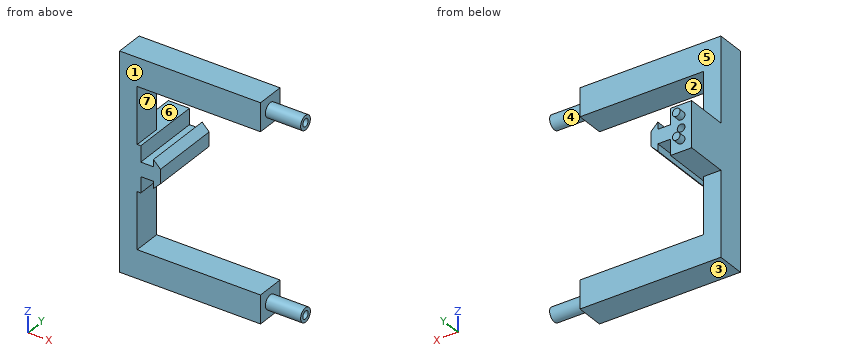
Autodesk Inventor part; units mm, degrees
ref_plane "YZ Plane" through (0, 0, 0) normal (1, 0, 0) x (0, 1, 0)
ref_plane "XZ Plane" through (0, 0, 0) normal (0, 1, 0) x (-1, 0, 0)
ref_plane "XY Plane" through (0, 0, 0) normal (0, 0, 1) x (1, 0, 0)
sketch "Sketch1" plane through (0, 0, 0) normal (0, 1, 0) x (-1, 0, 0)
  line L0 (0, 0) -> (7.62, 0)
  line L1 (7.62, 0) -> (7.62, -16.51)
  line L2 (7.62, -16.51) -> (0, -16.51)
  line L3 (0, -16.51) -> (0, 0)
  line L4 (0, 0) -> (0, -5.715)
  line L5 (0, -5.715) -> (-7.112, -5.715)
  line L6 (-7.112, -5.715) -> (-7.112, -10.795)
  line L7 (-7.112, -10.795) -> (0, -10.795)
  line L8 (-7.112, -5.715) -> (-4.572, -5.715)
  line L9 (-4.572, -5.715) -> (-4.572, -3.175)
  line L10 (-4.572, -3.175) -> (-7.112, -5.715)
  line L11 (-7.112, -10.795) -> (-4.572, -10.795)
  line L12 (-4.572, -10.795) -> (-4.572, -13.335)
  line L13 (-4.572, -13.335) -> (-7.112, -10.795)
  dimension "d0" = 7.62
  dimension "d1" = 16.51
  dimension "d2" = 5.715
  dimension "d3" = 7.112
  dimension "d4" = 5.08
  dimension "d5" = 2.54
  dimension "d6" = 2.54
  dimension "d7" = 2.54
extrude "Extrusion1" add sketch "Sketch1" along normal blind 25.4
sketch "Sketch2" plane through (0, 25.4, 0) normal (0, 1, 0) x (1, 0, 0)
  line L0 (-7.62, 0) -> (0, 0)
  line L1 (-3.81, 0) -> (-3.81, 4.064)
  line L2 (0, 16.51) -> (-7.62, 16.51)
  line L3 (-3.81, 16.51) -> (-3.81, 12.446)
  circle A0 centre (-3.81, 4.064) radius 1.397
  circle A1 centre (-3.81, 12.446) radius 1.397
  dimension "d10" = 4.064
  dimension "d11" = 4.064
  dimension "d12" = 2.794
  dimension "d13" = 2.794
extrude "Extrusion2" add sketch "Sketch2" along normal blind 2.54
sketch "Sketch3" plane through (0, 25.4, 0) normal (0, 1, 0) x (1, 0, 0)
  line L0 (-7.62, 0) -> (0, 0)
  line L1 (-3.81, 0) -> (-3.81, 8.255)
  dimension "d16" = 8.255
hole "Hole1" at (-3.81, 25.4, -8.255) direction (0, -1, 0) diameter 2.794 depth 11.43 tip angle 118
sketch "Sketch4" plane through (0, 0, -16.51) normal (0, 0, -1) x (-1, 0, 0)
  line L0 (7.62, 0) -> (0, 0)
  line L1 (7.62, 0) -> (1.27, 0)
  line L2 (1.27, 0) -> (1.27, 10.16)
  line L3 (1.27, 10.16) -> (7.62, 10.16)
  line L4 (7.62, 10.16) -> (7.62, 0)
  dimension "d24" = 6.35
  dimension "d25" = 10.16
extrude "Extrusion3" add sketch "Sketch4" along normal blind 30.48
sketch "Sketch5" plane through (-1.27, 0, -16.51) normal (1, 0, 0) x (0, 0, -1)
  line L0 (30.48, 10.16) -> (30.48, 0)
  line L1 (-16.51, 0) -> (30.48, 0)
  line L2 (30.48, 10.16) -> (20.32, 10.16)
  line L3 (20.32, 10.16) -> (20.32, 0)
  line L4 (20.32, 0) -> (30.48, 0)
  line L5 (30.48, 0) -> (30.48, 10.16)
  dimension "d28" = 10.16
extrude "Extrusion4" add sketch "Sketch5" along normal blind 44.45
sketch "Sketch6" plane through (43.18, 0, -16.51) normal (1, 0, 0) x (0, 0, -1)
  line L0 (30.48, 0) -> (30.48, 10.16)
  line L1 (30.48, 5.08) -> (25.4, 5.08)
  circle A0 centre (25.4, 5.08) radius 2.54
  point P0 (-16.51, 0)
  dimension "d31" = 5.08
  dimension "d32" = 5.08
extrude "Extrusion5" add sketch "Sketch6" along normal blind 12.7
sketch "Sketch7" plane through (55.88, 5.08, -41.91) normal (1, 0, 0) x (0, 0, -1)
  circle A0 centre (0, 0) radius 1.397
  point P0 (-41.91, -5.08)
  dimension "d35" = 2.794
hole "Hole2" at (55.88, 5.08, -41.91) direction (-1, 0, 0) diameter 2.794 depth 16.002 tip angle 118
sketch "Sketch8" plane through (-7.62, 0, 0) normal (0, 0, 1) x (1, 0, 0)
  line L0 (0, 0) -> (6.35, 0)
  line L1 (6.35, 0) -> (6.35, 10.16)
  line L2 (6.35, 10.16) -> (0, 10.16)
  line L3 (0, 10.16) -> (0, 0)
  point P0 (7.62, 0)
  dimension "d43" = 6.35
  dimension "d44" = 10.16
extrude "Extrusion6" add sketch "Sketch8" along normal blind 30.48
sketch "Sketch9" plane through (-1.27, 0, 0) normal (1, 0, 0) x (0, 0, -1)
  line L0 (-30.48, 0) -> (46.99, 0)
  line L1 (0, 10.16) -> (-30.48, 10.16)
  line L2 (-30.48, 0) -> (-20.32, 0)
  line L3 (-20.32, 0) -> (-20.32, 10.16)
  line L4 (-20.32, 10.16) -> (-30.48, 10.16)
  line L5 (-30.48, 10.16) -> (-30.48, 0)
  point P0 (0, 0)
  dimension "d47" = 10.16
extrude "Extrusion7" add sketch "Sketch9" along normal blind 44.45
sketch "Sketch10" plane through (43.18, 0, 0) normal (1, 0, 0) x (0, 0, -1)
  line L0 (-20.32, 10.16) -> (-20.32, 0)
  line L1 (-20.32, 5.08) -> (-25.4, 5.08)
  circle A0 centre (-25.4, 5.08) radius 2.54
  point P0 (0, 0)
  dimension "d50" = 5.08
  dimension "d51" = 5.08
extrude "Extrusion8" add sketch "Sketch10" along normal blind 12.7
sketch "Sketch11" plane through (55.88, 5.08, 25.4) normal (1, 0, 0) x (0, 0, -1)
  circle A0 centre (0, 0) radius 1.397
  point P0 (25.4, -5.08)
  dimension "d54" = 2.794
hole "Hole3" at (55.88, 5.08, 25.4) direction (-1, 0, 0) diameter 2.794 depth 16.002 tip angle 118
properties part number "Grab Rail v2"
CAD build for the part. Positions are in the model's coordinates, mm. Face numbers are marked on the shaded views. A direction names the side the tool comes from. Coordinates: 2 decimals unless noted, no trailing zeros. Loops run counter-clockwise (first coordinate to the right, second up) from the corner with the lowest first, then second, coordinate; pieces in that order, holes last. Notation, with made-up numbers: (6, 13.25) -> (47, 13.25) arc R21 cw to (47, 41.25) -> close; hole circle Ø4 at (78, 50). An arc over 180 degrees is marked (long way). One line per item, written item: value.
1. Slice it at B-B on y = 21. Write the cut outline in (x, z) (3 decimals), and give its area (3 significant figures).
Answers:
outline: (-7.62, -16.51) -> (0, -16.51) -> (0, -10.795) -> (4.572, -10.795) -> (4.572, -13.335) -> (7.112, -10.795) -> (7.112, -5.715) -> (4.572, -3.175) -> (4.572, -5.715) -> (0, -5.715) -> (0, 0) -> (-7.62, 0) -> close; hole circle Ø2.794 at (-3.81, -8.255)
area: 162 mm^2
2. Flat gauge pins, fed straight in: P1, Ø4.5, axis at y = 9.5, z = -15, coming from the +X side; P2, Ø5, axis at y = 4, z = -25.5, coming from the +X side; P3, Ø2.5, axis at x = -3, y = 13.5, coming from the +Z side. Where does each tip first touch, or does it go through?
Answers:
P1: stops at x = 5.16
P2: stops at x = -1.27
P3: stops at z = 0
3. Slice it at C-C on x = 15. Write the cut outline in (y, z), and give its area (3 significant figures).
Answers:
outline: (0, -46.99) -> (10.16, -46.99) -> (10.16, -36.83) -> (0, -36.83) -> close; (0, 20.32) -> (10.16, 20.32) -> (10.16, 30.48) -> (0, 30.48) -> close
area: 206 mm^2
4. Pull direction Z, two halves, no side cores. Call the marked faces 1, 2, 3 and 4: pulls with the +Z half, pulls with the -Z half, needs draft (parallel to the pull), parting line crosses it, or undercut.
Answers:
face 1: needs draft
face 2: undercut
face 3: pulls with the -Z half
face 4: undercut
5. Slice it at D-D on z = 12.5. Write the cut outline in (x, y).
Answers:
outline: (-7.62, 0) -> (-1.27, 0) -> (-1.27, 10.16) -> (-7.62, 10.16) -> close
6. Drill centre lines: line 1 (Z direction, x = -3.81, y = 19.5); line 2 (Z direction, x = 28.5, y = 2); line 3 (X direction, y = 16.25, z = -15). Where is each one in solid material? Low to high. Write a range as [from, to].
Answers:
line 1: z = [-16.51, -9.65], [-6.86, 0]
line 2: z = [-46.99, -36.83], [20.32, 30.48]
line 3: x = [-7.62, 0]
7. Which spindle directions (+Z, -Z, +X, -X, +Y, -Y) get a long thin tool onto all of the face, cutting with end or side? Do the marked faces 5, 6 and 7. Say none if no direction does.
Answers:
face 5: +Z, +X, -X, +Y
face 6: +X, +Y
face 7: +X, +Y, -Y
8. Slice it at A-A on x = 42. Write the cut outline in (y, z), and give its area (3 significant figures).
Answers:
outline: (0, -46.99) -> (10.16, -46.99) -> (10.16, -36.83) -> (0, -36.83) -> close; (0, 20.32) -> (10.16, 20.32) -> (10.16, 30.48) -> (0, 30.48) -> close; hole circle Ø2.79 at (5.08, -41.91); hole circle Ø2.79 at (5.08, 25.4)
area: 194 mm^2
